Work out the finished part from the listing and answer in its coordinate system (mm). A direction names the side the tool comes from. Round coordinates to 2 decimals unless told otherwise and drop trailing zeros. Write each loop counter-clockwise with the first axis right and the second up, starting at its lowest first coordinate (ties: lowest second). Pieces come first, ordered by that corner, then holes. Notation, with made-up numbers: (74, -10.5) -> (132, -10.5) arc R17 ccw to (132, 11.5) -> close; hole circle Ø7 at (31.25, 21). An arc over 180 degrees is marked (long way). One line per item, written item: value.
```python
from build123d import *

# Parameters (mm, degrees)
SKETCH_1_R                = 1.6
EXTRUDE_1_DEPTH           = 2
EXTRUDE_START             = 2
EXTRUDE_2_OUTLINE_R       = 1.6
EXTRUDE_2_DEPTH           = 2
EXTRUDE_START_2           = 4
SKETCH_1_4_R              = 1.6
EXTRUDE_3_DEPTH           = 3
FILLET_2_DEPTH            = 4
FILLET_2_2_DEPTH          = 2
FILLET_3_DEPTH            = 2
EXTRUDE_4_DEPTH           = 7
EXTRUDE_5_DEPTH           = 2
SKETCH_4_W                = 10
SKETCH_4_H                = 15
EXTRUDE_6_DEPTH           = 7
CUT_EXTRUDE_START         = -2
SKETCH_5_W                = 10
SKETCH_5_H                = 7
SKETCH_5_W_2              = 7.6
SKETCH_5_H_2              = 4.6
CUT_EXTRUDE_1_DEPTH       = 2.5
CUT_EXTRUDE_START_2       = -5
CUT_EXTRUDE_2_OUTLINE_W   = 2.5
CUT_EXTRUDE_2_OUTLINE_H   = 1.2
CUT_EXTRUDE_2_DEPTH       = 10
CUT_EXTRUDE_2_2_OUTLINE_W = 2.5
CUT_EXTRUDE_2_2_OUTLINE_H = 4.6
CUT_EXTRUDE_2_2_DEPTH     = 1.2
CUT_EXTRUDE_START_3       = 3.8
CUT_EXTRUDE_2_3_OUTLINE_W = 2.5
CUT_EXTRUDE_2_3_OUTLINE_H = 4.6
CUT_EXTRUDE_2_3_DEPTH     = 1.2
FILLET_4_R                = 5
FILLET_5_R                = 1
FILLET_6_R                = 0.5
SKETCH_6_R                = 2.1
CUT_EXTRUDE_3_DEPTH       = 4


with BuildPart() as part:
    # Эскиз1 → Бобышка-Вытянуть1 (new body)
    with BuildSketch(Plane.XY):
        with BuildLine():
            ThreePointArc((12.207759872, -13.227645252), (18.328207768, -18.328207768), (13.227645252, -12.207759872))
            ThreePointArc((13.227645252, -12.207759872), (16.629831585, -6.888301783), (17.985547445, -0.721167868))
            ThreePointArc((17.985547445, -0.721167868), (25.92, 0), (17.985547445, 0.721167868))
            ThreePointArc((17.985547445, 0.721167868), (15.70130603, 8.801646945), (10, 14.966629547))
            Line((10, 14.966629547), (10, 27))
            Line((10, 27), (-10, 27))
            Line((-10, 27), (-10, 14.966629547))
            ThreePointArc((-10, 14.966629547), (-11.137870812, 14.140291149), (-12.207759872, 13.227645252))
            ThreePointArc((-12.207759872, 13.227645252), (-18.328207768, 18.328207768), (-13.227645252, 12.207759872))
            ThreePointArc((-13.227645252, 12.207759872), (-16.629831585, 6.888301783), (-17.985547445, 0.721167868))
            ThreePointArc((-17.985547445, 0.721167868), (-25.92, 0), (-17.985547445, -0.721167868))
            ThreePointArc((-17.985547445, -0.721167868), (-6.888301783, -16.629831585), (12.207759872, -13.227645252))
        make_face()
        with Locations((15.499780644, -15.499780644)):
            Circle(SKETCH_1_R, mode=Mode.SUBTRACT)
        with Locations((-21.92, 0)):
            Circle(SKETCH_1_R, mode=Mode.SUBTRACT)
        with Locations((21.92, 0)):
            Circle(SKETCH_1_R, mode=Mode.SUBTRACT)
        with Locations((-15.499780644, 15.499780644)):
            Circle(SKETCH_1_R, mode=Mode.SUBTRACT)
    extrude(amount=EXTRUDE_1_DEPTH)

    # Бобышка-Вытянуть2: read off the stored shape, not the designer's step
    # Бобышка-Вытянуть2 outline → Бобышка-Вытянуть2 (add)
    with BuildSketch(Plane.XY.offset(EXTRUDE_START)):
        with BuildLine():
            ThreePointArc((17.985547445, -0.721167868), (25.92, 0), (17.985547445, 0.721167868))
            ThreePointArc((17.985547445, 0.721167868), (15.70130603, 8.801646944), (10, 14.966629547))
            Line((10, 14.966629547), (10, 27))
            Line((10, 27), (-10, 27))
            Line((-10, 27), (-10, 14.966629547))
            ThreePointArc((-10, 14.966629547), (-15.70130603, 8.801646944), (-17.985547445, 0.721167868))
            ThreePointArc((-17.985547445, 0.721167868), (-25.92, 0), (-17.985547445, -0.721167868))
            ThreePointArc((-17.985547445, -0.721167868), (0, -18), (17.985547445, -0.721167868))
        make_face()
        with Locations((-21.92, 0)):
            Circle(EXTRUDE_2_OUTLINE_R, mode=Mode.SUBTRACT)
        with Locations((21.92, 0)):
            Circle(EXTRUDE_2_OUTLINE_R, mode=Mode.SUBTRACT)
    extrude(amount=EXTRUDE_2_DEPTH)

    # Эскиз1<4> → Бобышка-Вытянуть3 (add)
    # profile 1 of 3: a face of its own
    with BuildSketch(Plane.XY.offset(EXTRUDE_START_2)):
        with BuildLine():
            ThreePointArc((17.985547445, 0.721167868), (17.996386499, 0.360656336), (18, 0))
            ThreePointArc((18, 0), (17.996386499, -0.360656336), (17.985547445, -0.721167868))
            ThreePointArc((17.985547445, -0.721167868), (25.92, 0), (17.985547445, 0.721167868))
        make_face()
        with Locations((21.92, 0)):
            Circle(SKETCH_1_4_R, mode=Mode.SUBTRACT)
    # profile 2 of 3: a face of its own
    with BuildSketch(Plane.XY.offset(EXTRUDE_START_2)):
        with BuildLine():
            ThreePointArc((-10, 14.966629547), (0, 18), (10, 14.966629547))
            Line((10, 14.966629547), (10, 27))
            Line((10, 27), (-10, 27))
            Line((-10, 27), (-10, 14.966629547))
        make_face()
    # profile 3 of 3: a face of its own
    with BuildSketch(Plane.XY.offset(EXTRUDE_START_2)):
        with BuildLine():
            ThreePointArc((-17.985547445, -0.721167868), (-17.996386499, -0.360656336), (-18, 0))
            ThreePointArc((-18, 0), (-17.996386499, 0.360656336), (-17.985547445, 0.721167868))
            ThreePointArc((-17.985547445, 0.721167868), (-25.92, 0), (-17.985547445, -0.721167868))
        make_face()
        with Locations((-21.92, 0)):
            Circle(SKETCH_1_4_R, mode=Mode.SUBTRACT)
    extrude(amount=EXTRUDE_3_DEPTH)

    # Скругление2: read off the stored shape, not the designer's step
    # Скругление2 outline → Скругление2 (add)
    with BuildSketch(Plane.XY):
        with BuildLine():
            ThreePointArc((-16.805693431, 6.447376855), (-18.568168191, 4.400080171), (-21.230145985, 3.940063634))
            ThreePointArc((-21.230145985, 3.940063634), (-19.102842691, 2.839652215), (-17.985547445, 0.721167868))
            ThreePointArc((-17.985547445, 0.721167868), (-17.629661873, 3.632495318), (-16.805693431, 6.447376855))
        make_face()
        with BuildLine():
            ThreePointArc((-21.230145985, -3.940063634), (-18.568168191, -4.400080171), (-16.805693431, -6.447376855))
            ThreePointArc((-16.805693431, -6.447376855), (-17.629661873, -3.632495318), (-17.985547445, -0.721167868))
            ThreePointArc((-17.985547445, -0.721167868), (-19.102842691, -2.839652215), (-21.230145985, -3.940063634))
        make_face()
        with BuildLine():
            ThreePointArc((17.985547445, 0.721167868), (19.102842691, 2.839652215), (21.230145985, 3.940063634))
            ThreePointArc((21.230145985, 3.940063634), (18.568168191, 4.400080171), (16.805693431, 6.447376855))
            ThreePointArc((16.805693431, 6.447376855), (17.629661873, 3.632495318), (17.985547445, 0.721167868))
        make_face()
        with BuildLine():
            ThreePointArc((17.985547445, -0.721167868), (17.629661873, -3.632495318), (16.805693431, -6.447376855))
            ThreePointArc((16.805693431, -6.447376855), (18.568168191, -4.400080171), (21.230145985, -3.940063634))
            ThreePointArc((21.230145985, -3.940063634), (19.102842691, -2.839652215), (17.985547445, -0.721167868))
        make_face()
    extrude(amount=FILLET_2_DEPTH)

    # Fillet 2 2 outline → Fillet 2 2 (add)
    with BuildSketch(Plane.XY):
        with BuildLine():
            ThreePointArc((-17.798025906, 12.225934478), (-16.241004168, 10.018351115), (-16.442403683, 7.324435892))
            ThreePointArc((-16.442403683, 7.324435892), (-15.034615533, 9.897491388), (-13.227645252, 12.207759872))
            ThreePointArc((-13.227645252, 12.207759872), (-15.515686945, 11.49981227), (-17.798025906, 12.225934478))
        make_face()
        with BuildLine():
            ThreePointArc((7.324435892, -16.442403683), (10.018351115, -16.241004168), (12.225934478, -17.798025906))
            ThreePointArc((12.225934478, -17.798025906), (11.49981227, -15.515686945), (12.207759872, -13.227645252))
            ThreePointArc((12.207759872, -13.227645252), (9.897491388, -15.034615533), (7.324435892, -16.442403683))
        make_face()
        with BuildLine():
            ThreePointArc((13.227645252, -12.207759872), (15.515686945, -11.49981227), (17.798025906, -12.225934478))
            ThreePointArc((17.798025906, -12.225934478), (16.241004168, -10.018351115), (16.442403683, -7.324435892))
            ThreePointArc((16.442403683, -7.324435892), (15.034615533, -9.897491388), (13.227645252, -12.207759872))
        make_face()
    extrude(amount=FILLET_2_2_DEPTH)

    # Скругление3: read off the stored shape, not the designer's step
    # Скругление3 outline → Скругление3 (add)
    with BuildSketch(Plane.XY):
        with BuildLine():
            Line((-10, 14.966629547), (-10, 17.679682972))
            ThreePointArc((-10, 17.679682972), (-10.776344158, 16.70501479), (-11.899956129, 17.243702506))
            ThreePointArc((-11.899956129, 17.243702506), (-11.511477517, 15.194104067), (-12.207759872, 13.227645252))
            ThreePointArc((-12.207759872, 13.227645252), (-11.137870812, 14.140291149), (-10, 14.966629547))
        make_face()
    extrude(amount=FILLET_3_DEPTH)

    # Эскиз2 → Бобышка-Вытянуть4 (add)
    with BuildSketch(Plane.XY.offset(7)):
        with BuildLine():
            Line((-10, 27), (-8, 27))
            Line((-8, 27), (-8, 16.124515497))
            ThreePointArc((-8, 16.124515497), (-9.018601608, 15.577702816), (-10, 14.966629547))
            Line((-10, 14.966629547), (-10, 27))
        make_face()
        with BuildLine():
            Line((10, 27), (8, 27))
            Line((8, 27), (8, 16.124515497))
            ThreePointArc((8, 16.124515497), (9.018601608, 15.577702816), (10, 14.966629547))
            Line((10, 14.966629547), (10, 27))
        make_face()
    extrude(amount=EXTRUDE_4_DEPTH)

    # Эскиз3 → Бобышка-Вытянуть5 (add)
    with BuildSketch(Plane.XY.offset(14)):
        with BuildLine():
            Line((10, 27), (-8, 27))
            Line((-8, 27), (-8, 16.124515497))
            ThreePointArc((-8, 16.124515497), (1.155497714, 17.962873518), (10, 14.966629547))
            Line((10, 14.966629547), (10, 27))
        make_face()
        with BuildLine():
            Line((-8, 27), (-10, 27))
            Line((-10, 27), (-10, 14.966629547))
            ThreePointArc((-10, 14.966629547), (-9.018601608, 15.577702816), (-8, 16.124515497))
            Line((-8, 16.124515497), (-8, 27))
        make_face()
    extrude(amount=EXTRUDE_5_DEPTH)

    # Эскиз4 → Бобышка-Вытянуть6 (add)
    with BuildSketch(Plane(origin=(0, 0, 0), x_dir=(-1, 0, 0), z_dir=(0, 0, -1))):
        with Locations((0, 34.5)):
            Rectangle(SKETCH_4_W, SKETCH_4_H)
    extrude(amount=-EXTRUDE_6_DEPTH)

    # Эскиз5 → Вырез-Вытянуть1 (cut)
    with BuildSketch(Plane(origin=(0, 42, 0), x_dir=(1, 0, 0), z_dir=(0, 1, 0)).offset(CUT_EXTRUDE_START)):
        with Locations((0, -3.5)):
            Rectangle(SKETCH_5_W, SKETCH_5_H)
        with Locations((0, -3.5)):
            Rectangle(SKETCH_5_W_2, SKETCH_5_H_2, mode=Mode.SUBTRACT)
    extrude(amount=-CUT_EXTRUDE_1_DEPTH, mode=Mode.SUBTRACT)

    # Вырез-Вытянуть2: read off the stored shape, not the designer's step
    # Вырез-Вытянуть2 outline → Вырез-Вытянуть2 (cut)
    with BuildSketch(Plane.YZ.offset(CUT_EXTRUDE_START_2)):
        with Locations((32.75, 6.4)):
            Rectangle(CUT_EXTRUDE_2_OUTLINE_W, CUT_EXTRUDE_2_OUTLINE_H)
        with Locations((32.75, 0.6)):
            Rectangle(CUT_EXTRUDE_2_OUTLINE_W, CUT_EXTRUDE_2_OUTLINE_H)
    extrude(amount=CUT_EXTRUDE_2_DEPTH, mode=Mode.SUBTRACT)

    # Cut-Extrude 2 2 outline → Cut-Extrude 2 2 (cut)
    with BuildSketch(Plane.YZ.offset(CUT_EXTRUDE_START_2)):
        with Locations((32.75, 3.5)):
            Rectangle(CUT_EXTRUDE_2_2_OUTLINE_W, CUT_EXTRUDE_2_2_OUTLINE_H)
    extrude(amount=CUT_EXTRUDE_2_2_DEPTH, mode=Mode.SUBTRACT)

    # Cut-Extrude 2 3 outline → Cut-Extrude 2 3 (cut)
    with BuildSketch(Plane.YZ.offset(CUT_EXTRUDE_START_3)):
        with Locations((32.75, 3.5)):
            Rectangle(CUT_EXTRUDE_2_3_OUTLINE_W, CUT_EXTRUDE_2_3_OUTLINE_H)
    extrude(amount=CUT_EXTRUDE_2_3_DEPTH, mode=Mode.SUBTRACT)

    # Скругление4
    fillet_4_edges = [part.edges().sort_by_distance(p)[0] for p in [
        (10, 14.966629547, 1),
    ]]
    fillet(fillet_4_edges, radius=FILLET_4_R)

    # Скругление5
    fillet_5_edges = [part.edges().sort_by_distance(p)[0] for p in [
        (-10, 14.966629547, 3),
        (-10, 27, 8),
        (10, 27, 8),
    ]]
    fillet(fillet_5_edges, radius=FILLET_5_R)

    # Скругление6
    fillet_6_edges = [part.edges().sort_by_distance(p)[0] for p in [
        (5, 41, 0),
        (-5, 29.25, 0),
        (-5, 29.25, 7),
        (5, 41, 7),
        (5, 35.75, 7),
        (5, 35.75, 0),
        (-5, 41, 7),
        (-5, 41, 0),
        (3.8, 38.75, 5.8),
        (-3.8, 38.75, 5.8),
        (-3.8, 38.75, 1.2),
        (3.8, 38.75, 1.2),
        (5, 29.25, 0),
        (5, 29.25, 7),
        (-5, 35.75, 7),
        (-5, 35.75, 0),
        (3.8, 32.75, 5.8),
        (-3.8, 32.75, 5.8),
        (-3.8, 32.75, 1.2),
        (3.8, 32.75, 1.2),
    ]]
    fillet(fillet_6_edges, radius=FILLET_6_R)

    # Эскиз6 → Вырез-Вытянуть3 (cut)
    with BuildSketch(Plane(origin=(0, 0, 0), x_dir=(-1, 0, 0), z_dir=(0, 0, -1))):
        with Locations((-21.92, 0)):
            Circle(SKETCH_6_R)
        with Locations((21.92, 0)):
            Circle(SKETCH_6_R)
    extrude(amount=-CUT_EXTRUDE_3_DEPTH, mode=Mode.SUBTRACT)


solid = part.part
```
(1) Find section C-C on x = 21.92. Give the vertices of the cut face in (y, z).
Reported:
outline: (-4, 0) -> (-2.1, 0) -> (-2.1, 4) -> (-1.6, 4) -> (-1.6, 7) -> (-4, 7) -> close; (1.6, 4) -> (2.1, 4) -> (2.1, 0) -> (4, 0) -> (4, 7) -> (1.6, 7) -> close
(2) Find section B-B on y = 23. Give the vertices of the cut face in (x, z).
Reported:
outline: (-10, 0) -> (10, 0) -> (10, 16) -> (-10, 16) -> close; hole (-8, 7) -> (8, 7) -> (8, 14) -> (-8, 14) -> close
(3) For a pull along X with two mould halves and no side action, classify faces 1 (the face through (8, 22, 10)), 2 (the face through (-3.8, 39, 4)), 3 (the face through (0, 36, 0)), 4 (the face through (-10.8, 16.7, 1)) as pulls with the +X half, pulls with the -X half, needs draft (parallel to the pull), parting line crosses it, or undercut.
Reported:
face 1: undercut
face 2: pulls with the -X half
face 3: needs draft
face 4: undercut
(4) Find section A-A on z = 11.75. Give the vertices of the cut face in (x, y), plus the area to 3 significant figures.
Reported:
outline: (-10, 14.97) arc R18 cw to (-8, 16.12) -> (-8, 27) -> (-9, 27) arc R1 ccw to (-10, 26) -> close; (8, 16.12) arc R18 cw to (10, 14.97) -> (10, 26) arc R1 ccw to (9, 27) -> (8, 27) -> close
area: 45.3 mm2
(5) A tool of negligible diameter and unlimited length cuts with its end or side. For faces 5 (the face through (0, 39, 1.2)), 6 (the face through (0, 22, 14)), 7 (the face through (0, 39, 5.8)), 8 (the face through (0, 40, 1)), 9 (the face through (3.8, 39, 4)), from which of +Z, -Z, +X, -X, +Y, -Y can it reach the whole face along a straight path? Write none if from no direction.
Reported:
face 5: -Z, +X, -X
face 6: +Y, -Y
face 7: +Z, +X, -X
face 8: none
face 9: +Z, -Z, +X
(6) Consider probe 1 along X at (y, z) = (26, 10); probe 2 along Y at (x, z) = (-21.92, 5.75); probe 3 along X at (y, z) = (0.5, 4.5). Determine where each line is inside the solid, lowest interval first.
Reported:
probe 1: x = -10 to -8, 8 to 10
probe 2: y = -4 to -1.6, 1.6 to 4
probe 3: x = -25.89 to -23.44, -20.4 to -17.99, 17.99 to 20.4, 23.44 to 25.89
(7) Find section D-D on y = -3. Give the vertices of the cut face in (x, z).
Reported:
outline: (-24.57, 0) -> (24.57, 0) -> (24.57, 7) -> (19.27, 7) -> (19.27, 4) -> (-19.27, 4) -> (-19.27, 7) -> (-24.57, 7) -> close
(8) Flat-ended cylindrical pins translate along their axes: pin 1 Ø3.5 at (y, z) = (30, 3.5) entering from +X; pin 2 Ø3.5 at (x, z) = (1, 5) entering from -Y; pin 3 Ø11 at (x, y) = (6, -8.5) entering from +Z; pin 4 Ø1 at (x, z) = (2, 13) entering from -Y. Find the tip coordinate at first contact, or state that the pin passes through.
Reported:
pin 1: stops at x = 5
pin 2: stops at y = -18
pin 3: stops at z = 4
pin 4: passes through
